Source: CAD feature listing. Evaluate the final solid. Frame: model axes, mm. Face numbers are marked on the shaded views. Coordinates: 2 decimals unless noted, no trailing zeros. Order: outer loops, then holes, each group sorted by start corner. A loop starts at its lowest first (then second) coordinate and runs counter-clockwise, first axis right, second up.
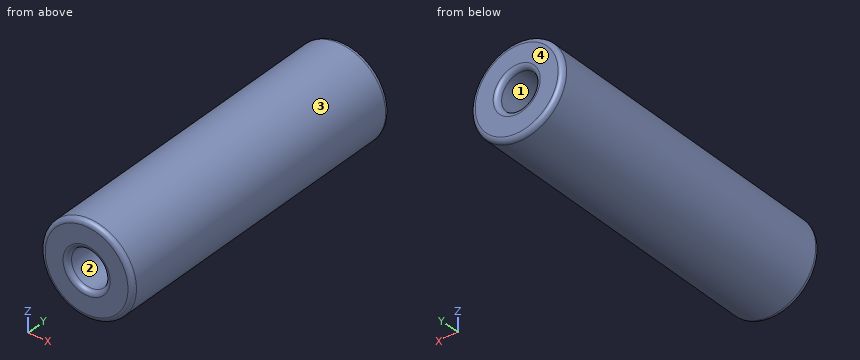
```python
from build123d import *

# Parameters (mm, degrees)
FILLET_R = 1


with BuildPart() as part:
    # Sketch → Revolution (revolve)
    with BuildSketch(Plane.XY):
        Polygon((4, 68), (9.8, 68), (9.8, 0), (4, 0), (4, 10), (0, 10), (0, 58), (4, 58), align=None)
    revolve(axis=Axis((0, 0, 0), (0, 1, 0)))

    # Fillet
    fillet_edges = [part.edges().sort_by_distance(p)[0] for p in [
        (-4, 0, 0),
        (-9.8, 0, 0),
        (-9.8, 68, 0),
        (-4, 68, 0),
    ]]
    fillet(fillet_edges, radius=FILLET_R)


solid = part.part
```
1. Contact query for flat-ended pins moving along their axis: P1, Ø2.5, axis at x = 2, z = -1.5, coming from the -Y side; P2, Ø4, axis at y = 10.5, z = 5.5, coming from the -X side; P3, Ø7, axis at x = 0, z = 0, coming from the +Y side. Output: stop coordinate, or through.
2. Draft query along Z for the marked faces 1, 2, 3 and 4. Return one class per face: +Z half, -Z half, draft (parallel to the pull), parting line (faces both ways), or undercut.
3. Section query A-A, the plane z = 0. Output: boundary loops of the cut face in (x, y).
4. Section query C-C, the plane x = 0. Output: boundary loops of the cut face in (y, z).
5. Section query B-B, the plane y = 7.5. Output: boundary loops of the cut face in (x, z).
6. Material intervals for line 1 along X through (y, z) = (60.25, 0); line 2 along Z through (x, y) = (-0.5, 55), sorted ascending.
Answer key:
1. P1: stops at y = 10
1. P2: stops at x = -9.15
1. P3: stops at y = 58
2. face 1: undercut
2. face 2: undercut
2. face 3: parting line
2. face 4: draft
3. outline: (-9.8, 1) arc R1 ccw to (-8.8, 0) - (-5, 0) arc R1 ccw to (-4, 1) - (-4, 10) - (4, 10) - (4, 1) arc R1 ccw to (5, 0) - (8.8, 0) arc R1 ccw to (9.8, 1) - (9.8, 67) arc R1 ccw to (8.8, 68) - (5, 68) arc R1 ccw to (4, 67) - (4, 58) - (-4, 58) - (-4, 67) arc R1 ccw to (-5, 68) - (-8.8, 68) arc R1 ccw to (-9.8, 67) - close
4. outline: (0, -8.8) arc R1 ccw to (1, -9.8) - (67, -9.8) arc R1 ccw to (68, -8.8) - (68, -5) arc R1 ccw to (67, -4) - (58, -4) - (58, 4) - (67, 4) arc R1 ccw to (68, 5) - (68, 8.8) arc R1 ccw to (67, 9.8) - (1, 9.8) arc R1 ccw to (0, 8.8) - (0, 5) arc R1 ccw to (1, 4) - (10, 4) - (10, -4) - (1, -4) arc R1 ccw to (0, -5) - close
5. outline: circle Ø19.6 at (0, 0); hole circle Ø8 at (0, 0)
6. line 1: x = -9.8 to -4, 4 to 9.8
6. line 2: z = -9.79 to 9.79
